Verification items for the finished model (mm, model axes). Face numbers are marked on the shaded views. Coordinates: 2 decimals unless noted, no trailing zeros. Order: outer loops, then holes, each group sorted by start corner. A loop starts at its lowest first (then second) coordinate and runs counter-clockwise, first axis right, second up. Notation, with made-up numbers: (-1.5, 44) -> (36.5, 44) arc R28 cw to (36.5, 69) -> close; hole circle Ø9 at (-31.75, -17). An arc over 180 degrees is marked (long way). Answer as CSV lines item,"result".
```python
from build123d import *

# Parameters (mm, degrees)
SCHIZZO1_W                   = 13
SCHIZZO1_H                   = 3.57
ESTRUSIONE_ESTRUSIONE1_DEPTH = 6
SCHIZZO3_W                   = 3.3
SCHIZZO3_H                   = 0.5
ESTRUSIONE_ESTRUSIONE2_DEPTH = 2
RACCORDO1_R                  = 0.1
SCHIZZO4_W                   = 1
SCHIZZO4_H                   = 1
TAGLIO_ESTRUSIONE1_DEPTH     = 7
SCHIZZO5_W                   = 1.001424396
SCHIZZO5_H                   = 3
ESTRUSIONE_ESTRUSIONE3_DEPTH = 0.5
RACCORDO2_R                  = 0.3
ESTRUSIONE_ESTRUSIONE4_DEPTH = 4
TAGLIO_ESTRUSIONE2_DEPTH     = 0.3


with BuildPart() as part:
    # Schizzo1 → Estrusione-Estrusione1 (new body)
    with BuildSketch(Plane.XY):
        Rectangle(SCHIZZO1_W, SCHIZZO1_H)
    extrude(amount=ESTRUSIONE_ESTRUSIONE1_DEPTH)

    # Schizzo3 → Estrusione-Estrusione2 (add)
    with BuildSketch(Plane.XZ.offset(1.785)):
        with Locations((0, 5.75)):
            Rectangle(SCHIZZO3_W, SCHIZZO3_H)
        with Locations((0, 0.25)):
            Rectangle(SCHIZZO3_W, SCHIZZO3_H)
    extrude(amount=ESTRUSIONE_ESTRUSIONE2_DEPTH)

    # Raccordo1
    raccordo1_edges = [part.edges().sort_by_distance(p)[0] for p in [
        (1.65, -3.785, 0.25),
        (-1.65, -3.785, 0.25),
        (-1.65, -3.785, 5.75),
        (1.65, -3.785, 5.75),
        (-1.65, -1.785, 0.25),
        (1.65, -1.785, 0.25),
        (-1.65, -1.785, 5.75),
        (1.65, -1.785, 5.75),
    ]]
    fillet(raccordo1_edges, radius=RACCORDO1_R)

    # Schizzo4 → Taglio-Estrusione1 (cut, through all)
    with BuildSketch(Plane.XY.offset(6)):
        with Locations((0, -2.485)):
            Rectangle(SCHIZZO4_W, SCHIZZO4_H)
    extrude(amount=-TAGLIO_ESTRUSIONE1_DEPTH, mode=Mode.SUBTRACT)

    # Schizzo5 → Estrusione-Estrusione3 (add)
    with BuildSketch(Plane(origin=(0, 1.785, 0), x_dir=(1, 0, 0), z_dir=(0, 1, 0))):
        with Locations((-2.499287802, -3)):
            Rectangle(SCHIZZO5_W, SCHIZZO5_H)
    extrude(amount=ESTRUSIONE_ESTRUSIONE3_DEPTH)

    # Raccordo2
    raccordo2_edges = [part.edges().sort_by_distance(p)[0] for p in [
        (-3, 2.285, 3),
        (-1.998575604, 2.285, 3),
    ]]
    fillet(raccordo2_edges, radius=RACCORDO2_R)

    # Schizzo7 → Estrusione-Estrusione4 (add)
    with BuildSketch(Plane.XY.offset(5)):
        Polygon((-5.428309071, 1.15280402), (7.290989084, 6.916004863), (7.167174091, 7.189262704), (-5.552124064, 1.42606186), align=None)
    extrude(amount=-ESTRUSIONE_ESTRUSIONE4_DEPTH)

    # Schizzo8 → Taglio-Estrusione2 (cut)
    with BuildSketch(Plane(origin=(-1.481816175, 3.270346158, 0), x_dir=(0.910859468, 0.412716645, 0), z_dir=(-0.412716645, 0.910859468, 0))):
        with BuildLine():
            Line((-3.598949006, -2.25), (4.101050994, -2.25))
            ThreePointArc((4.101050994, -2.25), (4.454604385, -2.396446609), (4.601050994, -2.75))
            Line((4.601050994, -2.75), (4.601050994, -3.25))
            ThreePointArc((4.601050994, -3.25), (4.454604385, -3.603553391), (4.101050994, -3.75))
            Line((4.101050994, -3.75), (-3.598949006, -3.75))
            Line((-3.598949006, -3.75), (-3.598949006, -2.25))
        make_face()
    extrude(amount=-TAGLIO_ESTRUSIONE2_DEPTH, mode=Mode.SUBTRACT)


solid = part.part
```
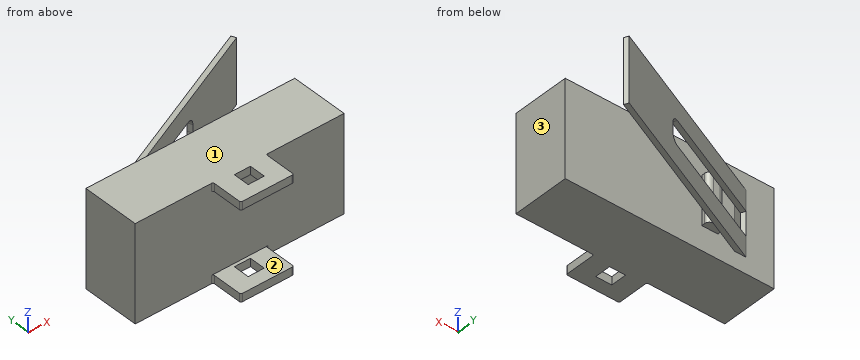
Item 1: Section check D-D, the plane x = -2.5. Record the boundary of the cut face in (y, z) (3 decimals), plus the area to 3 significant figures.
Answer list:
outline,"(-1.785, 0) -> (1.785, 0) -> (1.785, 1.5) -> (2.285, 1.5) -> (2.285, 4.5) -> (1.785, 4.5) -> (1.785, 6) -> (-1.785, 6) -> close; (2.48, 1) -> (2.809, 1) -> (2.809, 2.25) -> (2.48, 2.25) -> close; (2.48, 3.75) -> (2.809, 3.75) -> (2.809, 5) -> (2.48, 5) -> close"
area,"23.7 mm2"
Item 2: Section check B-B, the plane z = 4.2. Record the boundary of the cut face in (x, y) (3 decimals), plus the area to 3 significant figures.
Answer list:
outline,"(-6.5, -1.785) -> (6.5, -1.785) -> (6.5, 1.785) -> (-1.999, 1.785) -> (-1.999, 1.985) arc R0.3 ccw to (-2.299, 2.285) -> (-2.7, 2.285) arc R0.3 ccw to (-3, 1.985) -> (-3, 1.785) -> (-4.033, 1.785) -> (7.291, 6.916) -> (7.167, 7.189) -> (-4.76, 1.785) -> (-6.5, 1.785) -> close"
area,"50.7 mm2"
Item 3: Section check A-A, the plane x = 6. Record the boundary of the cut face in (y, z) (3 decimals), plus the area to 3 significant figures.
Answer list:
outline,"(-1.785, 0) -> (1.785, 0) -> (1.785, 6) -> (-1.785, 6) -> close; (6.331, 1) -> (6.66, 1) -> (6.66, 5) -> (6.331, 5) -> close"
area,"22.7 mm2"
Item 4: Thickness scan on line 1 (Y direction, x = -1, z = 0.65) (3 decimals); line 2 (Z direction, x = 1.5, y = -2); line 3 (Z direction, x = 0.25, y = 4). Record the ranges inside material, lowest first.
Answer list:
line 1,"-1.785 to 1.785"
line 2,"0 to 0.5, 5.5 to 6"
line 3,"1 to 2.25, 3.75 to 5"
Item 5: Depth check by flat-ended pin: pin 1 Ø3 at (x, z) = (3, 4) entering from +Y; pin 2 Ø1 at (x, y) = (-1, 4) entering from -Z; pin 3 Ø3 at (x, y) = (-1, 3.5) entering from +Z. Enter the tip coordinate at first touch or a pass-through.
Answer list:
pin 1,"y = 5.98"
pin 2,"z = 1"
pin 3,"z = 5"
Item 6: Section check C-C, the plane y = 3. Record the boundary of the cut face in (x, z).
Answer list:
outline,"(-2.08, 1) -> (-1.35, 1) -> (-1.35, 2.25) -> (-2.08, 2.25) -> close; (-2.08, 3.75) -> (-1.35, 3.75) -> (-1.35, 5) -> (-2.08, 5) -> close"
Item 7: Release check for a two-part mould opening along Z. For the marked faces 1, 2 and 3 record: +Z half, -Z half, draft (parallel to the pull), parting line (faces both ways), or undercut.
Answer list:
face 1,"+Z half"
face 2,"undercut"
face 3,"draft"
